Work out the finished part from the listing and answer in its coordinate system (mm). Face numbers are marked on the shaded views. A direction names the side the tool comes from. Coordinates: 2 decimals unless noted, no trailing zeros. Write each loop counter-clockwise with the first axis right and the second up, starting at its lowest first coordinate (ties: lowest second). Pieces come first, ordered by that corner, then holes. Notation, with made-up numbers: (33, -18.75) - (74, -18.75) arc R19 cw to (74, 2.25) - close; hole circle Ø1 at (88, -35.5). An arc over 180 degrees is marked (long way). Use a Markdown table: item, result. Add a question column.
(1) Find the intervals of material crossed by line 1 (X direction, y = 26.25, z = 0); line 2 (Z direction, x = 7.5, y = -25); line 3 (X direction, y = 23.5, z = -1.5), in increasing order. Write a range as from..to.
(2) The part is cut by section B-B, the plane z = 0. State how many separate pieces and enclosed holes the cut face has, then the cut area to 3 significant figures.
(3) Given pin 1 Ø2 at (x, z) = (18.5, 3) entering from -Y; pin 2 Ø3 at (y, z) = (-7, 1) entering from -X; pin 3 Ø4.5 at (y, z) = (-26.5, -1) entering from -X, each flat-ended and moving along its own axis, determine where each tip first touches the part or whether it passes through.
(4) For a pull along Y with two mould halves and no side action, classify the marked faces 3, 4, 5 and 6 as released by +Y, released by -Y, zero draft, split by the parting line, or undercut.
(5) A tool of negligible diameter and unlimited length cuts with its end or side. For the marked faces 1 and 2, from which of +Z, -Z, +X, -X, +Y, -Y can it reach the whole face along a straight path? Write none if from no direction.
(6) The part is cut by section A-A, the plane x = 6. Give the vertices of the cut face in (y, z), then the cut area to 3 significant figures.
(7) The part is cut by section C-C, the plane y = -25. Give the vertices of the cut face in (x, z).
(8) The part is cut by section D-D, the plane x = 25. Give the vertices of the cut face in (y, z), then the cut area to 3 significant figures.
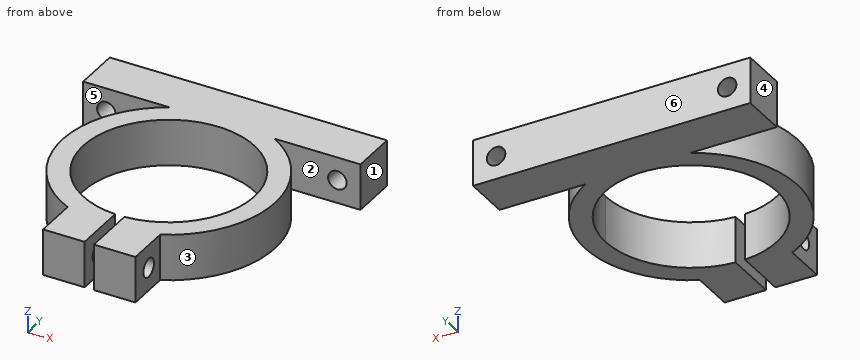
from build123d import *

# Parameters (mm, degrees)
CYLINDER002_R     = 2
CYLINDER002_DEPTH = 10
CYLINDER001_R     = 18.5
CYLINDER001_DEPTH = 10
CYLINDER004_R     = 2
CYLINDER004_DEPTH = 20
BOX002_W          = 2
BOX002_H          = 15
BOX002_DEPTH      = 10
CYLINDER003_R     = 2
CYLINDER003_DEPTH = 10
BOX_W             = 60
BOX_H             = 10
BOX_DEPTH         = 10
BOX001_W          = 20
BOX001_H          = 10
BOX001_DEPTH      = 10
CYLINDER_R        = 23
CYLINDER_DEPTH    = 10


with BuildPart() as cylinder002:
    # Cylinder002 → Cylinder002 (new body)
    with BuildSketch(Plane(origin=(25, 20, 0), x_dir=(1, 0, 0), z_dir=(0, 1, 0))):
        Circle(CYLINDER002_R)
    extrude(amount=CYLINDER002_DEPTH)


with BuildPart() as cylinder001:
    # Cylinder001 → Cylinder001 (new body)
    with BuildSketch(Plane.XY.offset(-5)):
        Circle(CYLINDER001_R)
    extrude(amount=CYLINDER001_DEPTH)


with BuildPart() as cylinder004:
    # Cylinder004 → Cylinder004 (new body)
    with BuildSketch(Plane(origin=(-10, -25, 0), x_dir=(0, 0, -1), z_dir=(1, 0, 0))):
        Circle(CYLINDER004_R)
    extrude(amount=CYLINDER004_DEPTH)


with BuildPart() as cube002:
    # Box002 → Box002 (new body)
    with BuildSketch(Plane(origin=(-1, -30, -5), x_dir=(1, 0, 0), z_dir=(0, 0, 1))):
        with Locations((1, 7.5)):
            Rectangle(BOX002_W, BOX002_H)
    extrude(amount=BOX002_DEPTH)


with BuildPart() as negative_fusion:
    # Cylinder003 → Cylinder003 (new body)
    with BuildSketch(Plane(origin=(-25, 20, 0), x_dir=(1, 0, 0), z_dir=(0, 1, 0))):
        Circle(CYLINDER003_R)
    extrude(amount=CYLINDER003_DEPTH)

    # Fusion001: union Cylinder002, Cylinder001, Cylinder004, Cube002
    add(cylinder002.part)
    add(cylinder001.part)
    add(cylinder004.part)
    add(cube002.part)


with BuildPart() as cube:
    # Box → Box (new body)
    with BuildSketch(Plane(origin=(-30, 20, -5), x_dir=(1, 0, 0), z_dir=(0, 0, 1))):
        with Locations((30, 5)):
            Rectangle(BOX_W, BOX_H)
    extrude(amount=BOX_DEPTH)


with BuildPart() as cube001:
    # Box001 → Box001 (new body)
    with BuildSketch(Plane(origin=(-10, -30, -5), x_dir=(1, 0, 0), z_dir=(0, 0, 1))):
        with Locations((10, 5)):
            Rectangle(BOX001_W, BOX001_H)
    extrude(amount=BOX001_DEPTH)


with BuildPart() as cut:
    # Cylinder → Cylinder (new body)
    with BuildSketch(Plane.XY.offset(-5)):
        Circle(CYLINDER_R)
    extrude(amount=CYLINDER_DEPTH)

    # Fusion: union Cube, Cube001
    add(cube.part)
    add(cube001.part)

    # Cut: cut Negative Fusion
    add(negative_fusion.part, mode=Mode.SUBTRACT)


solid = cut.part
Model answer:
| question | item | result |
|---|---|---|
| 1 | line 1 | -30..-27, -23..23, 27..30 |
| 1 | line 2 | -5..-2, 2..5 |
| 1 | line 3 | -30..-26.32, -23.68..23.68, 26.32..30 |
| 2 | separate pieces | 5 |
| 2 | enclosed holes | 0 |
| 2 | area | 1,120 mm^2 |
| 3 | pin 1 | y = -14.92 |
| 3 | pin 2 | x = -22.33 |
| 3 | pin 3 | x = -10 |
| 4 | face 3 | undercut |
| 4 | face 4 | zero draft |
| 4 | face 5 | undercut |
| 4 | face 6 | released by +Y |
| 5 | face 1 | +Z, -Z, +X, +Y, -Y |
| 5 | face 2 | +Z, -Z, +X |
| 6 | outline | (-30, -5) - (-17.5, -5) - (-17.5, 5) - (-30, 5) - close; (17.5, -5) - (30, -5) - (30, 5) - (17.5, 5) - close; hole circle Ø4 at (-25, 0) |
| 6 | area | 237 mm^2 |
| 7 | outline | (-10, -5) - (-1, -5) - (-1, -2) - (-10, -2) - close; (-10, 2) - (-1, 2) - (-1, 5) - (-10, 5) - close; (1, -5) - (10, -5) - (10, -2) - (1, -2) - close; (1, 2) - (10, 2) - (10, 5) - (1, 5) - close |
| 8 | outline | (20, -5) - (30, -5) - (30, -2) - (20, -2) - close; (20, 2) - (30, 2) - (30, 5) - (20, 5) - close |
| 8 | area | 60.0 mm^2 |
